CAD build for the part. Positions are in the model's coordinates, mm. A direction names the side the tool comes from. Round coordinates to 2 decimals unless told otherwise and drop trailing zeros. Order: outer loops, then holes, each group sorted by start corner. A loop starts at its lowest first (then second) coordinate and runs counter-clockwise, first axis right, second up.
```python
from build123d import *

# Parameters (mm, degrees)
SKETCH1_R               = 65
SKETCH1_R_2             = 1
BOSS_EXTRUDE1_DEPTH     = 1
CUT_EXTRUDE1_DEPTH      = 1
CUT_EXTRUDE2_DEPTH      = 1
CUT_EXTRUDE2_DEPTH_BACK = 92.929320676
SKETCH3_R               = 4.5


with BuildPart() as part:
    # Sketch1 → Boss-Extrude1 (new, symmetric)
    with BuildSketch(Plane(origin=(0, 0, 0), x_dir=(1, 0, 0), z_dir=(0, 1, 0))):
        with Locations(Location((0, 0, 0), (0, 0, 270))):
            Circle(SKETCH1_R)
        with Locations(Location((0, 0, 0), (0, 0, 270))):
            Circle(SKETCH1_R_2, mode=Mode.SUBTRACT)
    extrude(amount=BOSS_EXTRUDE1_DEPTH, both=True)

    # Sketch2 → Cut-Extrude1 (cut)
    with BuildSketch(Plane(origin=(0, 1, 0), x_dir=(1, 0, 0), z_dir=(0, 1, 0))):
        Polygon((67.534801337, -30.330981694), (7.5, 4.330127019), (7.5, 73.652344444), (-7.5, 73.652344444), (-7.5, 4.330127019), (-67.534801337, -30.330981694), (-60.034801337, -43.32136275), (0, -8.660254038), (60.034801337, -43.32136275), align=None)
    extrude(amount=-CUT_EXTRUDE1_DEPTH, mode=Mode.SUBTRACT)

    # Sketch3 → Cut-Extrude2 (cut, two sides: drawn at the far end of the back side and taken through both)
    with BuildSketch(Plane(origin=(0, 0, 0), x_dir=(1, 0, 0), z_dir=(0, 1, 0)).offset(-CUT_EXTRUDE2_DEPTH_BACK)):
        with Locations(Location((41.13620668, 23.75, 0), (0, 0, 270))):
            Circle(SKETCH3_R)
        with Locations(Location((0, -47.5, 0), (0, 0, 270))):
            Circle(SKETCH3_R)
        with Locations(Location((-41.13620668, 23.75, 0), (0, 0, 270))):
            Circle(SKETCH3_R)
    extrude(amount=CUT_EXTRUDE2_DEPTH + CUT_EXTRUDE2_DEPTH_BACK, mode=Mode.SUBTRACT)


solid = part.part
```
1. Tool access for faces 1 (the face through (1, -1, -1)), 2 (the face through (-33.22, 0.51, 10.52)): list every direction of +Z, -Z, +X, -X, +Y, -Y with a clear straight run to the whole face (end or side of a thin tool).
2. Pin check, flat tip, straight feed: P1, Ø0.8, axis at y = 0.5, z = -32.5, coming from the +X side. Stop position of the tip, or through.
3. Cut at C-C, the plane z = 47.5. Write the cut outline in (x, y).
4. Cut at A-A, the plane y = 0.4. Write the cut outline in (x, z), and give its area (3 significant figures).
5. Cut at B-B, the plane z = -23.75. Write the cut outline in (x, y), and give its area (3 significant figures).
6. Mould opens along Z. For faces 3 (the face through (19.52, 0.01, 62)), 4 (the face through (25.7, 0.5, 23.5)), 5 (the face through (37, 1, -20)) say: released by +Z, released by -Z, zero draft, split by the parting line, or undercut.
7. Drill centre lines: line 1 (Z direction, x = 0, y = -0.75); line 2 (X direction, y = -0.25, z = 0); line 3 (X direction, y = 0.65, z = -24). Where is each one in solid material? Low to high.
8. Cut at D-D, the plane x = 27.5. Write the cut outline in (y, z).
Outcome:
1. face 1: +Z, -Z, +X, -X, -Y
1. face 2: +Y
2. P1: stops at x = 56.52
3. outline: (-44.37, -1) - (-4.5, -1) - (-4.5, 1) - (-44.37, 1) - close; (4.5, -1) - (44.37, -1) - (44.37, 1) - (4.5, 1) - close
4. outline: (-59.67, 25.79) arc R65 ccw to (-7.5, -64.57) - (-7.5, -4.33) - close; (-52.17, 38.78) - (0, 8.66) - (52.17, 38.78) arc R65 ccw to start; (7.5, -64.57) arc R65 ccw to (59.67, 25.79) - (7.5, -4.33) - close; hole circle Ø9 at (-41.14, -23.75); hole circle Ø9 at (0, 47.5); hole circle Ø9 at (41.14, -23.75)
4. area: 10,300 mm2
5. outline: (-60.51, -1) - (-45.64, -1) - (-45.64, 1) - (-60.51, 1) - close; (-36.64, -1) - (36.64, -1) - (36.64, 1) - (7.5, 1) - (7.5, 0) - (-7.5, 0) - (-7.5, 1) - (-36.64, 1) - close; (45.64, -1) - (60.51, -1) - (60.51, 1) - (45.64, 1) - close
5. area: 191 mm2
6. face 3: split by the parting line
6. face 4: undercut
6. face 5: zero draft
7. line 1: z = -65 to -1, 1 to 43, 52 to 65
7. line 2: x = -65 to -1, 1 to 65
7. line 3: x = -60.41 to -45.63, -36.64 to -7.5, 7.5 to 36.64, 45.63 to 60.41
8. outline: (-1, -58.9) - (1, -58.9) - (1, 7.22) - (0, 7.22) - (0, 24.54) - (1, 24.54) - (1, 58.9) - (-1, 58.9) - close
